Input: part model. Units: mm. Frame: model coordinates. A direction names the side the tool comes from. Give positions to 0.01 mm unless a question says otherwise; leave off trailing zeros. Loops run counter-clockwise (first coordinate to the right, second up) from the corner with the lowest first, then second, coordinate; pieces in that order, holes last. Notation, with made-up numbers: M 27.25,85.25 L 46.25,85.25 A22 ccw 46.25,91.25 Z; hole C 15,43.25 d5. An arc over 180 degrees is marked long. One line per item, written item: value. Start each with the question number.
(1) Section A-A on y = 7. Output: boundary loops of the cut face in (x, z).
(2) Pull-direction query (X, two-part tool) for faces 1 (the flat face through (-2, 31, 9.25)), 2 (the cylindrical face through (-3.25, 29.34, 15.08)), 3 (the flat face through (47.5, 29, 10)); classes: released by +X, released by -X, zero draft, split by the parting line, or undercut.
(3) Pin query (flat end, axial travel): P1, Ø2, axis at x = 42.5, z = 10.5, coming from the +Y side; P2, Ø10, axis at y = 12, z = 15.5, coming from the -X side; P3, Ø1, axis at x = 28, z = 2, coming from the +Y side. Return the tip coordinate at first contact, or that it passes through.
(4) Access query for faces 4 (the flat face through (-3, 29, 1)), 5 (the cylindrical face through (8.64, 43.27, 7.13)), 6 (the flat face through (42, 31, 9.25)), 7 (the flat face through (-2, 31, 10.75)). Directions: +Z, -Z, +X, -X, +Y, -Y. A direction counts if a zero-diameter tool reaches every point of the face in a straight line with its end or side. Return the directions, or none.
(5) Section B-B on x = 8. Output: boundary loops of the cut face in (y, z), plus the area to 3 significant figures.
(6) Section C-C on x = 26. Output: boundary loops of the cut face in (y, z).
(7) Ray query, line 1 along Z through (x, y) = (45.5, 29.25); line 2 along Z through (x, y) = (-5, 29); line 3 along X through (y, z) = (17, 16.75). Return the intervals inside material, ascending. Write a range as from..to.
```python
from build123d import *

# Parameters (mm, degrees)
SALIENTE_EXTRUIR1_DEPTH = 20
REDONDEO1_R             = 1
CROQUIS2_R              = 8
SALIENTE_EXTRUIR2_DEPTH = 6
SALIENTE_EXTRUIR2_DRAFT = -18
CROQUIS3_R              = 2.94
SALIENTE_EXTRUIR3_DEPTH = 3.6
SALIENTE_EXTRUIR4_DEPTH = 2.7
SALIENTE_EXTRUIR5_DEPTH = 0.75


with BuildPart() as part:
    # Croquis1 → Saliente-Extruir1 (new body)
    with BuildSketch(Plane.XY):
        Polygon((40, 0), (0, 0), (0, 35.5), (8.658841891, 40.499184697), (37.668841891, 40.499184697), (40, 35.5), align=None)
    extrude(amount=SALIENTE_EXTRUIR1_DEPTH)

    # Redondeo1
    redondeo1_edges = [part.edges().sort_by_distance(p)[0] for p in [
        (40, 17.75, 20),
        (0, 17.75, 20),
        (40, 17.75, 0),
        (0, 17.75, 0),
    ]]
    fillet(redondeo1_edges, radius=REDONDEO1_R)


with BuildPart() as saliente_extruir2_tool:
    # Croquis2 → Saliente-Extruir2 (with draft: the straight prism first)
    with BuildSketch(Plane(origin=(0, 35.5, 0), x_dir=(-1, 0, 0), z_dir=(0, -1, 0))):
        with Locations((-8, -10)):
            Circle(CROQUIS2_R)
    extrude(amount=-SALIENTE_EXTRUIR2_DEPTH)
    # Saliente-Extruir2: the draft: its side faces are tilted about the plane it starts from
    saliente_extruir2_sides = [saliente_extruir2_tool.faces().sort_by_distance(p)[0] for p in [
        (16, 38.5, 10),
    ]]
    draft(saliente_extruir2_sides, Plane(origin=(0, 35.5, 0), x_dir=(-1, 0, 0), z_dir=(0, -1, 0)), SALIENTE_EXTRUIR2_DRAFT)


with BuildPart() as part_1:
    add(part.part)

    # Saliente-Extruir2: add saliente_extruir2_tool
    add(saliente_extruir2_tool.part)

    # Croquis3 → Saliente-Extruir3 (add)
    with BuildSketch(Plane(origin=(0, 41.5, 0), x_dir=(1, 0, 0), z_dir=(0, 1, 0))):
        with Locations(Location((8, -10, 0), (0, 0, 180))):
            Circle(CROQUIS3_R)
    extrude(amount=SALIENTE_EXTRUIR3_DEPTH)

    # Croquis4 → Saliente-Extruir4 (add)
    with BuildSketch(Plane(origin=(0, 28.01, 0), x_dir=(-1, 0, 0), z_dir=(0, -1, 0))):
        with BuildLine():
            Line((-45, -19), (-40, -19))
            Line((-40, -19), (-40, -1))
            Line((-40, -1), (-45, -1))
            ThreePointArc((-45, -1), (-46.767766953, -1.732233047), (-47.5, -3.5))
            Line((-47.5, -3.5), (-47.5, -3.969223594))
            ThreePointArc((-47.5, -3.969223594), (-43.25, -5), (-47.5, -6.030776406))
            Line((-47.5, -6.030776406), (-47.5, -13.969223594))
            ThreePointArc((-47.5, -13.969223594), (-43.25, -15), (-47.5, -16.030776406))
            Line((-47.5, -16.030776406), (-47.5, -16.5))
            ThreePointArc((-47.5, -16.5), (-46.767766953, -18.267766953), (-45, -19))
        make_face()
        with BuildLine():
            Line((0, -19), (5, -19))
            ThreePointArc((5, -19), (6.767766953, -18.267766953), (7.5, -16.5))
            Line((7.5, -16.5), (7.5, -16.030776406))
            ThreePointArc((7.5, -16.030776406), (3.25, -15), (7.5, -13.969223594))
            Line((7.5, -13.969223594), (7.5, -6.030776406))
            ThreePointArc((7.5, -6.030776406), (3.25, -5), (7.5, -3.969223594))
            Line((7.5, -3.969223594), (7.5, -3.5))
            ThreePointArc((7.5, -3.5), (6.767766953, -1.732233047), (5, -1))
            Line((5, -1), (0, -1))
            Line((0, -1), (0, -19))
        make_face()
    extrude(amount=-SALIENTE_EXTRUIR4_DEPTH)

    # Croquis5 → Saliente-Extruir5 (add, symmetric)
    with BuildSketch(Plane.XY.offset(10)):
        Polygon((-6, 31.21), (-1.000247602, 31.91), (0, 31.91), (0, 30.71), (-6, 30.71), align=None)
        Polygon((40, 31.91), (41.000247602, 31.91), (46, 31.21), (46, 30.71), (40, 30.71), align=None)
    extrude(amount=SALIENTE_EXTRUIR5_DEPTH, both=True)


solid = part_1.part
```
Output values:
1. outline: M 0,1 A1 ccw 1,0 L 39,0 A1 ccw 40,1 L 40,19 A1 ccw 39,20 L 1,20 A1 ccw 0,19 Z
2. face 1: zero draft
2. face 2: undercut
2. face 3: released by +X
3. P1: stops at y = 31.84
3. P2: stops at x = 0
3. P3: stops at y = 40.5
4. face 4: -Z, -X, +Y, -Y
4. face 5: +Y
4. face 6: -Z, +X, +Y
4. face 7: +Z, -X, +Y
5. outline: M 0,0 L 40.12,0 L 40.12,3.5 L 41.5,3.95 L 41.5,7.06 L 45.1,7.06 L 45.1,12.94 L 41.5,12.94 L 41.5,16.05 L 40.12,16.5 L 40.12,20 L 0,20 Z
5. area: 841 mm²
6. outline: M 0,0 L 40.5,0 L 40.5,20 L 0,20 Z
7. line 1: z = 1.05..2.75, 7.25..12.75, 17.25..18.95
7. line 2: z = 1..2.81, 7.19..12.81, 17.19..19
7. line 3: x = 0..40
